Autodesk Inventor part; units mm, degrees
ref_plane "YZ Plane" through (0, 0, 0) normal (1, 0, 0) x (0, 1, 0)
ref_plane "XZ Plane" through (0, 0, 0) normal (0, 1, 0) x (-1, 0, 0)
ref_plane "XY Plane" through (0, 0, 0) normal (0, 0, 1) x (1, 0, 0)
sketch "Sketch1" plane through (0, 0, 0) normal (0, 0, 1) x (1, 0, 0)
  circle A0 centre (13, 8) radius 1.5
  circle A1 centre (13, 8) radius 1.5
  point P0 (0, 0)
  dimension "d0" = 3
extrude "Extrusion1" add sketch "Sketch1" along normal mid plane 10
sketch "Sketch2" plane through (13, 8, 5) normal (0, 0, 1) x (1, 0, 0)
  circle A0 centre (0, 0) radius 1.5
  circle A1 centre (0, 0) radius 3
  point P0 (-13, -8)
  dimension "d3" = 6
extrude "Extrusion2" add sketch "Sketch2" along normal blind 40 contours A0 | A1
chamfer "Chamfer1" distance 1 angle 45 1 edges at (10, 8, 45)
properties part number "wheel_pin_1"
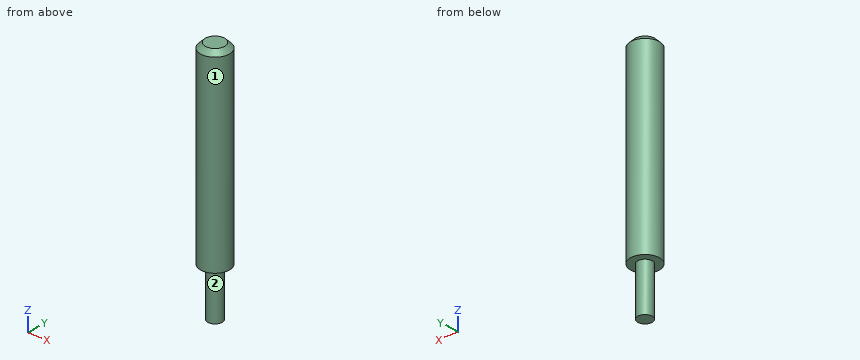
Verification items for the finished model (mm, model axes). Face numbers are marked on the shaded views. A direction names the side the tool comes from. Round coordinates to 2 decimals unless told otherwise and drop trailing zeros. Loops run counter-clockwise (first coordinate to the right, second up) from the corner with the lowest first, then second, coordinate; pieces in that order, holes last. Notation, with made-up numbers: (26, 63) -> (39, 63) arc R27 ccw to (39, 102) -> close; hole circle Ø6 at (-4, -2.5). An arc over 180 degrees is marked (long way). Answer as a JSON object with one key per item and string values.
Q1. Section check A-A (x = 13). Record the boundary of the cut face in (y, z), then the cut area to 3 significant figures.
Data:
{"outline": "(5, 5) -> (6.5, 5) -> (6.5, -5) -> (9.5, -5) -> (9.5, 5) -> (11, 5) -> (11, 44) -> (10, 45) -> (6, 45) -> (5, 44) -> close", "area": "269 mm2"}
Q2. Section check B-B (y = 8). Record the boundary of the cut face in (x, z), then the cut area to 3 significant figures.
Data:
{"outline": "(10, 5) -> (11.5, 5) -> (11.5, -5) -> (14.5, -5) -> (14.5, 5) -> (16, 5) -> (16, 44) -> (15, 45) -> (11, 45) -> (10, 44) -> close", "area": "269 mm2"}
Q3. Access from +Z, -Z, +X, -X, +Y, -Y to the whole of each face (thin tool, end or side, straight path). Record for the marked faces 1 and 2.
Data:
{"face 1": "+Z, -Z", "face 2": "-Z"}
Q4. Go/stop test with flat-tipped pins: P1, Ø2, axis at y = 10, z = 6, coming from the +X side; P2, Ø1, axis at y = 9.5, z = 3, coming from the -X side. Record where each tip stops, or that it passes through.
Data:
{"P1": "stops at x = 15.83", "P2": "stops at x = 11.88"}
Q5. Section check C-C (z = 19). Record the boundary of the cut face in (x, y), then the cut area to 3 significant figures.
Data:
{"outline": "circle Ø6 at (13, 8)", "area": "28.3 mm2"}
Q6. Scan lines: line 1 (X direction, y = 7.8, z = 41); line 2 (Z direction, x = 13.8, y = 9.3); line 3 (Y direction, x = 15.6, z = 22.5). Record each from-to range of solid material in increasing order. Write a range as from..to.
Data:
{"line 1": "x = 10.01..15.99", "line 2": "z = 5..45", "line 3": "y = 6.5..9.5"}
